Verification items for the finished model (mm, model axes). Face numbers are marked on the shaded views. A direction names the side the tool comes from. Round coordinates to 2 decimals unless told otherwise and drop trailing zeros. Order: outer loops, then holes, each group sorted by start corner. A loop starts at its lowest first (then second) coordinate and runs counter-clockwise, first axis right, second up. Notation, with made-up numbers: (89.25, 68) -> (108.25, 68) arc R6 ccw to (108.25, 78) -> close; hole circle Ø5 at (25.5, 40). An arc over 180 degrees is marked (long way). Put each result on its own line as item: value.
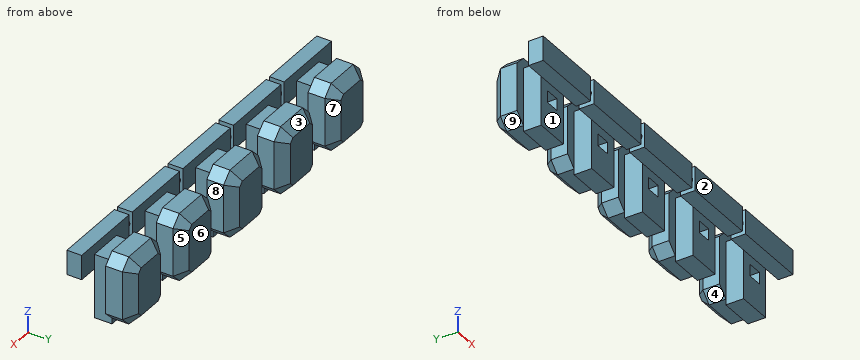
```python
from build123d import *

# Parameters (mm, degrees)
CYLINDER_R           = 0.5
CYLINDER_DEPTH       = 35
CYLINDER_PITCH_ANGLE = 90
SKETCH_W             = 3.5
SKETCH_H             = 6.5
PAD_DEPTH            = 1.8
PAD001_DEPTH         = 2.7
SKETCH002_W          = 1.5
SKETCH002_H          = 1.2
POCKET_DEPTH         = 2.5
SKETCH003_W          = 7.5
SKETCH003_H          = 2.5
PAD002_DEPTH         = 1.5
CHAMFER_SIZE         = 1
ARRAY_X_COUNT        = 5
ARRAY_X_PITCH        = 8


with BuildPart() as cylinder:
    # Cylinder → Cylinder (new body)
    with BuildSketch(Plane.XY):
        Circle(CYLINDER_R)
    extrude(amount=CYLINDER_DEPTH)


with BuildPart() as cylinder_1:
    # Cylinder pitch: moved
    add(cylinder.part.rotate(Axis((0, 0, 0), (0, 1, 0)), CYLINDER_PITCH_ANGLE))


with BuildPart() as cylinder_2:
    # Cylinder placement: moved
    add(cylinder_1.part.moved(Location((0, -2.55, 6.2))))


with BuildPart() as fusion:
    # Sketch → Pad (new body)
    with BuildSketch(Plane.XZ):
        with Locations((0, 3.25)):
            Rectangle(SKETCH_W, SKETCH_H)
    extrude(amount=PAD_DEPTH)

    # Sketch001 → Pad001 (new body)
    with BuildSketch(Plane(origin=(0, 0, 0), x_dir=(1, 0, 0), z_dir=(0, 1, 0))):
        Polygon((-1.75, -0.6), (1.75, -0.6), (2.75, -1.6), (2.75, -6.5), (1.75, -7.5), (-1.75, -7.5), (-2.75, -6.5), (-2.75, -1.6), align=None)
    extrude(amount=PAD001_DEPTH)

    # Sketch002 → Pocket (cut)
    with BuildSketch(Plane.XZ.offset(1.8)):
        with Locations((0, 3.5)):
            Rectangle(SKETCH002_W, SKETCH002_H)
    extrude(amount=-POCKET_DEPTH, mode=Mode.SUBTRACT)

    # Sketch003 → Pad002 (new body)
    with BuildSketch(Plane.XZ.offset(1.8)):
        with Locations((0, 6.25)):
            Rectangle(SKETCH003_W, SKETCH003_H)
    extrude(amount=PAD002_DEPTH)

    # Chamfer
    chamfer_edges = [fusion.edges().sort_by_distance(p)[0] for p in [
        (-2.75, 2.7, 4.05),
        (-2.25, 2.7, 1.1),
        (0, 2.7, 0.6),
        (2.25, 2.7, 1.1),
        (2.75, 2.7, 4.05),
        (2.25, 2.7, 7),
        (0, 2.7, 7.5),
        (-2.25, 2.7, 7),
    ]]
    chamfer(chamfer_edges, length=CHAMFER_SIZE)

    # Array X: Fusion ×5


with BuildPart() as fusion_1:
    add(fusion.part)
    with Locations(*[(i * ARRAY_X_PITCH, 0, 0) for i in range(1, ARRAY_X_COUNT)]):
        add(fusion.part)

    # Fusion: union Cylinder
    add(cylinder_2.part)


solid = fusion_1.part
```
Item 1: Sectioned sample at A-A, the plane y = -1.45. Give the number of separate pieces and of enclosed holes in the cut face, then the cut area to 3 significant figures.
Geometry check:
separate pieces: 5
enclosed holes: 5
area: 105 mm2
Item 2: Release check for a two-part mould opening along X. For the marked faces 6, 7, 8 and 9 record: pulls with the +X half, pulls with the -X half, needs draft (parallel to the pull), parting line crosses it, or undercut.
Geometry check:
face 6: needs draft
face 7: undercut
face 8: undercut
face 9: pulls with the -X half
Item 3: Sectioned sample at B-B, the plane x = 32. Record the boundary of the cut face in (y, z).
Geometry check:
outline: (-3.3, 5) -> (-1.8, 5) -> (-1.8, 4.1) -> (0.7, 4.1) -> (0.7, 2.9) -> (-1.8, 2.9) -> (-1.8, 0) -> (0, 0) -> (0, 0.6) -> (1.7, 0.6) -> (2.7, 1.6) -> (2.7, 6.5) -> (1.7, 7.5) -> (0, 7.5) -> (0, 6.5) -> (-1.8, 6.5) -> (-1.8, 7.5) -> (-3.3, 7.5) -> close
Item 4: Material ranges on line 1 along X through (y, z) = (2.1, 6); line 2 along Z through (x, y) = (0.5, -0.7); line 3 along X through (y, z) = (1.2, 7), recorded low to high.
Geometry check:
line 1: -2.35 to 2.35, 5.65 to 10.35, 13.65 to 18.35, 21.65 to 26.35, 29.65 to 34.35
line 2: 0 to 2.9, 4.1 to 6.5
line 3: -2.25 to 2.25, 5.75 to 10.25, 13.75 to 18.25, 21.75 to 26.25, 29.75 to 34.25
Item 5: Depth check by flat-ended pin: pin 1 Ø3 at (x, z) = (29, 1) entering from +Y; pin 2 Ø0.8 at (y, z) = (1, 4) entering from -X; pin 3 Ø1.6 at (x, z) = (9.5, 4.5) entering from -Y; pin 4 Ø1 at (x, z) = (18.5, 1.5) entering from -Y. Enter the tip coordinate at first touch or a pass-through.
Geometry check:
pin 1: y = 2.59
pin 2: x = -2.75
pin 3: y = -3.3
pin 4: y = 0
Item 6: Tool access check on the marked faces 1, 2, 3, 4 and 5. Record the directions out of +Z, -Z, +X, -X, +Y, -Y that give a thin tool (end or side, any length) a straight path to the whole face; none if there is none.
Geometry check:
face 1: -Z, +X, -X, -Y
face 2: +Z, -Z, +X, -X, -Y
face 3: +Z, +X, -X, +Y
face 4: -Z, +Y, -Y
face 5: +Z, -Z, +Y
